Input: part model. Units: mm. Frame: model coordinates. Face numbers are marked on the shaded views. Give positions to 0.01 mm unless a question says otherwise; leave off trailing zeros. Order: outer loops, then holes, each group sorted by start corner. A loop starts at its lowest first (then second) coordinate and runs counter-clockwise, first axis right, second up. Notation, with made-up numbers: M 29,-33.5 L 87,-33.5 A25 ccw 87,-17.5 Z; hole C 64.5,72 d2. An arc over 180 degrees is marked long. Use a Markdown table: item, result.
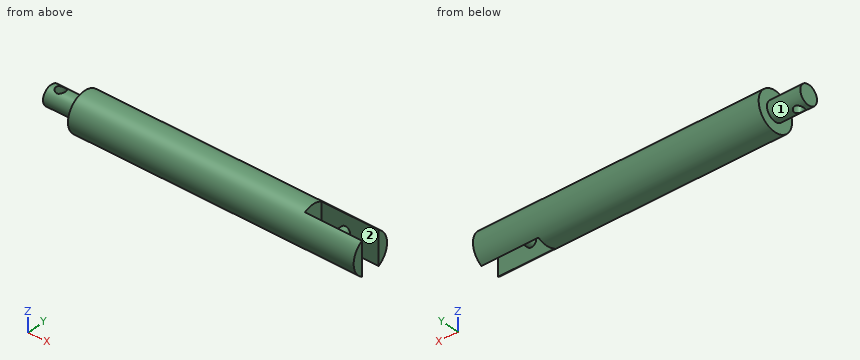
from build123d import *

# Parameters (mm, degrees)
SKETCH1_R           = 2
BOSS_EXTRUDE1_DEPTH = 7
SKETCH2_R           = 1
CUT_EXTRUDE1_DEPTH  = 4
SKETCH3_R           = 4
BOSS_EXTRUDE2_DEPTH = 60
SKETCH4_W           = 8.951999976
SKETCH4_H           = 4
CUT_EXTRUDE2_DEPTH  = 12
SKETCH5_R           = 1
BOSS_EXTRUDE3_DEPTH = 4


with BuildPart() as part:
    # Sketch1 → Boss-Extrude1 (new body)
    with BuildSketch(Plane(origin=(0, 0, 0), x_dir=(0, 0, -1), z_dir=(1, 0, 0))):
        Circle(SKETCH1_R)
    extrude(amount=BOSS_EXTRUDE1_DEPTH)

    # Sketch2 → Cut-Extrude1 (cut)
    with BuildSketch(Plane.XY.offset(2)):
        with Locations((2, 0)):
            Circle(SKETCH2_R)
    extrude(amount=-CUT_EXTRUDE1_DEPTH, mode=Mode.SUBTRACT)

    # Sketch3 → Boss-Extrude2 (add)
    with BuildSketch(Plane(origin=(7, 0, 0), x_dir=(0, 0, -1), z_dir=(1, 0, 0))):
        Circle(SKETCH3_R)
    extrude(amount=BOSS_EXTRUDE2_DEPTH)

    # Sketch4 → Cut-Extrude2 (cut)
    with BuildSketch(Plane(origin=(67, 0, 0), x_dir=(0, 0, -1), z_dir=(1, 0, 0))):
        with Locations((-0.118028397, 0)):
            Rectangle(SKETCH4_W, SKETCH4_H)
    extrude(amount=-CUT_EXTRUDE2_DEPTH, mode=Mode.SUBTRACT)

    # Sketch5 → Boss-Extrude3 (add)
    with BuildSketch(Plane(origin=(0, -2, 0), x_dir=(1, 0, 0), z_dir=(0, 1, 0))):
        with Locations(Location((60, 0, 0), (0, 0, 90))):
            Circle(SKETCH5_R)
    extrude(amount=BOSS_EXTRUDE3_DEPTH)


solid = part.part
1) Cut plane D-D on x = 2. Return loops of the section in (y, z).
Response values:
| item | result |
|---|---|
| outline | M -1,-1.73 L -1,1.73 A2 ccw Z; M 1,-1.73 A2 ccw 1,1.73 Z |
2) Cut plane C-C on x = 60. Return loops of the section in (y, z).
Response values:
| item | result |
|---|---|
| outline | M -2,-3.46 L -2,-1 L 2,-1 L 2,-3.46 A4 ccw 2,3.46 L 2,1 L -2,1 L -2,3.46 A4 ccw Z |
3) Cut plane B-B on z = 0. Return loops of the section in (x, y).
Response values:
| item | result |
|---|---|
| outline | M 0,-2 L 7,-2 L 7,-4 L 67,-4 L 67,-2 L 61,-2 L 61,2 L 67,2 L 67,4 L 7,4 L 7,2 L 0,2 Z; hole C 2,0 d2; hole M 55,-2 L 59,-2 L 59,2 L 55,2 Z |
4) Cut plane A-A on y = 0. Return loops of the section in (x, z).
Response values:
| item | result |
|---|---|
| outline | M 0,-2 L 1,-2 L 1,2 L 0,2 Z; M 3,-2 L 7,-2 L 7,-4 L 55,-4 L 55,4 L 7,4 L 7,2 L 3,2 Z; C 60,0 d2 |
5) Mould query, pull axis Y, two halves, no side actions, for the marked faces 1 and 2. Classes: released by +Y, released by -Y, zero draft, split by the parting line, or undercut.
Response values:
| item | result |
|---|---|
| face 1 | split by the parting line |
| face 2 | undercut |
6) First-contact query: pin 1 Ø3 at (x, y) = (2, 0) entering from -Z; pin 2 Ø3 at (x, y) = (14, -2) entering from +Z; pin 3 Ø2 at (y, z) = (3, 1.5) entering from -X. Flat tips, straight axial feed; report the tip coordinate or a pass-through.
Response values:
| item | result |
|---|---|
| pin 1 | stops at z = -2 |
| pin 2 | stops at z = 3.97 |
| pin 3 | stops at x = 7 |
7) Material intervals for line 1 (X direction, y = 0, z = 0); line 2 (Y direction, x = 2, z = 0.15); line 3 (Y direction, x = 60, z = -2), sorted ascending. Write a range as from..to.
Response values:
| item | result |
|---|---|
| line 1 | x = 0..1, 3..55, 59..61 |
| line 2 | y = -1.99..-1, 1..1.99 |
| line 3 | y = -3.46..-2, 2..3.46 |
